Part print with two shaded views. Sizes in mm from the minimum x, y, z corner. Round coordinates to 2 decimals unless told otherwise and drop trailing zeros. Order: outer loops, then holes, each group sorted by start corner. A loop starts at its lowest first (then second) coordinate and runs counter-clockwise, first axis right, second up. Notation, with made-up numbers: (74, 25) -> (85, 25) arc R22 ccw to (85, 37) -> close; hole circle Ø8 at (61.5, 9). An arc over 180 degrees is marked (long way). Put each result on its own line as item: value. Start each with the question number.
Q1. Cut at A-A, the plane z = 16.4. List the corners of the cut face in (x, y), and give its area (3 significant figures).
Q2. Cut at C-C, the plane x = 16.4. List the corners of the cut face in (y, z), and give its area (3 significant figures).
Q3. Cut at B-B, the plane x = 44. List the corners of the cut face in (y, z).
Q4. Probe L1, parallel to X at y = 1.4, z = 8; L2, parallel to Z at x = 16.4, y = 3.65. List the from-to ranges inside material, lowest first.
Q5. Cut at D-D, the plane y = 3.1. State how many separate pieces and enclosed holes the cut face has, and give its area (3 significant figures).
Q6. Flat gauge pin, fed straight in: P1, Ø4.5, axis at x = 63.6, z = 16.4, coming from the -Y side. Where does the tip first touch, or does it go through?
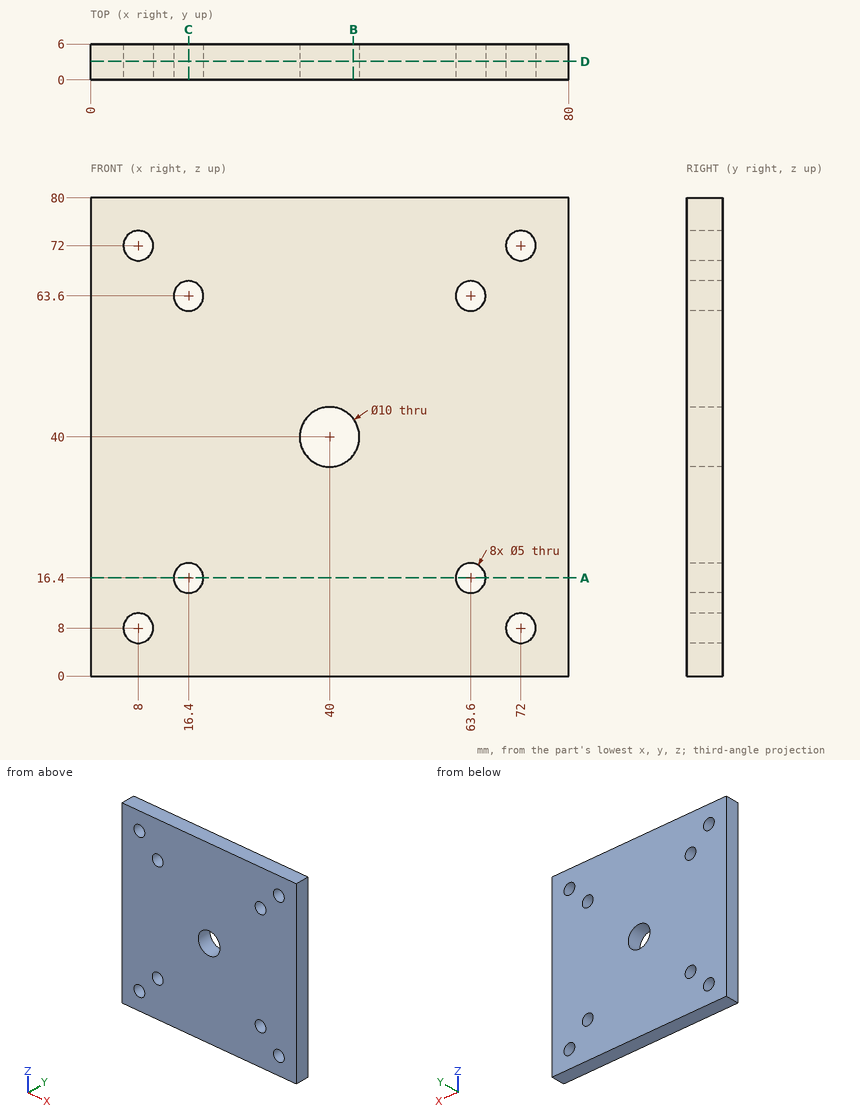
Ans:
1. outline: (0, 0) -> (13.9, 0) -> (13.9, 6) -> (0, 6) -> close; (18.9, 0) -> (61.1, 0) -> (61.1, 6) -> (18.9, 6) -> close; (66.1, 0) -> (80, 0) -> (80, 6) -> (66.1, 6) -> close
1. area: 420 mm^2
2. outline: (0, 0) -> (6, 0) -> (6, 13.9) -> (0, 13.9) -> close; (0, 18.9) -> (6, 18.9) -> (6, 61.1) -> (0, 61.1) -> close; (0, 66.1) -> (6, 66.1) -> (6, 80) -> (0, 80) -> close
2. area: 420 mm^2
3. outline: (0, 0) -> (6, 0) -> (6, 37) -> (0, 37) -> close; (0, 43) -> (6, 43) -> (6, 80) -> (0, 80) -> close
4. L1: x = 0 to 5.5, 10.5 to 69.5, 74.5 to 80
4. L2: z = 0 to 13.9, 18.9 to 61.1, 66.1 to 80
5. separate pieces: 1
5. enclosed holes: 9
5. area: 6,160 mm^2
6. P1: passes through
